Work out the finished part from the listing and answer in its coordinate system (mm). Face numbers are marked on the shaded views. A direction names the side the tool comes from. Round coordinates to 2 decimals unless told otherwise and drop trailing zeros. Order: outer loops, then holes, each group sorted by start corner. A loop starts at its lowest first (then second) coordinate and runs counter-clockwise, first axis right, second up. Notation, with made-up numbers: (3.5, 15.5) - (26.5, 15.5) arc R21 cw to (26.5, 52.5) - close; hole circle Ø10 at (22, 85). An arc over 180 degrees is marked (long way). Answer in a Markdown table with one row per item.
from build123d import *

# Parameters (mm, degrees)
F1_DEPTH  = 6
F3_DEPTH  = 20
F5_DEPTH  = 40
F7_DEPTH  = 60
F9_DEPTH  = 2
F11_DEPTH = 2
F13_DEPTH = 2
F14_R     = 2.25
F15_DEPTH = 8
F16_R     = 2.25
F17_DEPTH = 8
F18_R     = 2.25
F19_DEPTH = 8
F20_R     = 3.75
F21_DEPTH = 2
F22_R     = 3.75
F23_DEPTH = 2
F24_R     = 3.75
F25_DEPTH = 2
F26_SIZE  = 3
F27_W     = 20
F27_H     = 20
F28_DEPTH = 20


with BuildPart() as f1:
    # F0 (on Top) → F1 (new body)
    with BuildSketch(Plane.XY):
        Polygon((0, 66), (0, 0), (66, 0), (66, 26), (26, 26), (26, 66), align=None)
    extrude(amount=F1_DEPTH)

    # F2 (on face) → F3 (join)
    with BuildSketch(Plane.XY.offset(6)):
        Polygon((6, 66), (0, 66), (0, 0), (66, 0), (66, 6), (6, 6), align=None)
    extrude(amount=F3_DEPTH)

    # F4 (on face) → F5 (join)
    with BuildSketch(Plane.XY.offset(26)):
        Polygon((6, 6), (6, 26), (0, 26), (0, 0), (26, 0), (26, 6), align=None)
    extrude(amount=F5_DEPTH)

    # F6 (on face) → F7 (join)
    with BuildSketch(Plane.XY.offset(6)):
        Polygon((13.29, 6), (16, 6), (18.71, 6), (18.71, 8), (13.29, 8), align=None)
        Polygon((6, 18.71), (6, 16), (6, 13.29), (8, 13.29), (8, 18.71), align=None)
    extrude(amount=F7_DEPTH)

    # F8 (on face) → F9 (join)
    with BuildSketch(Plane.XY.offset(6)):
        Polygon((66, 13.29), (66, 16), (66, 18.71), (26, 18.71), (26, 13.29), align=None)
        Polygon((18.71, 66), (16, 66), (13.29, 66), (13.29, 26), (18.71, 26), align=None)
    extrude(amount=F9_DEPTH)

    # F10 (on face) → F11 (join)
    with BuildSketch(Plane(origin=(0, 6, 0), x_dir=(-1, 0, 0), z_dir=(0, 1, 0))):
        Polygon((-66, 18.71), (-66, 16), (-66, 13.29), (-26, 13.29), (-26, 16), (-26, 18.71), align=None)
    extrude(amount=F11_DEPTH)

    # F12 (on face) → F13 (join)
    with BuildSketch(Plane.YZ.offset(6)):
        Polygon((66, 13.29), (66, 16), (66, 18.71), (26, 18.71), (26, 13.29), align=None)
    extrude(amount=F13_DEPTH)

    # F14 (on face) → F15 (cut, through all)
    with BuildSketch(Plane.XZ):
        with Locations((56, 16)):
            Circle(F14_R)
        with Locations((16, 46)):
            Circle(F14_R)
        with Locations((36, 16)):
            Circle(F14_R)
    extrude(amount=-F15_DEPTH, mode=Mode.SUBTRACT)

    # F16 (on face) → F17 (cut, through all)
    with BuildSketch(Plane(origin=(0, 0, 0), x_dir=(0, -1, 0), z_dir=(-1, 0, 0))):
        with Locations((-16, 56)):
            Circle(F16_R)
        with Locations((-46, 16)):
            Circle(F16_R)
        with Locations((-16, 36)):
            Circle(F16_R)
    extrude(amount=-F17_DEPTH, mode=Mode.SUBTRACT)

    # F18 (on face) → F19 (cut, through all)
    with BuildSketch(Plane(origin=(0, 0, 0), x_dir=(1, 0, 0), z_dir=(0, 0, -1))):
        with Locations((46, -16)):
            Circle(F18_R)
        with Locations((16, -56)):
            Circle(F18_R)
        with Locations((16, -36)):
            Circle(F18_R)
    extrude(amount=-F19_DEPTH, mode=Mode.SUBTRACT)

    # F20 (on face) → F21 (cut)
    with BuildSketch(Plane.XZ):
        with Locations((16, 46)):
            Circle(F20_R)
        with Locations((36, 16)):
            Circle(F20_R)
        with Locations((56, 16)):
            Circle(F20_R)
    extrude(amount=-F21_DEPTH, mode=Mode.SUBTRACT)

    # F22 (on face) → F23 (cut)
    with BuildSketch(Plane(origin=(0, 0, 0), x_dir=(0, -1, 0), z_dir=(-1, 0, 0))):
        with Locations((-16, 56)):
            Circle(F22_R)
        with Locations((-46, 16)):
            Circle(F22_R)
        with Locations((-16, 36)):
            Circle(F22_R)
    extrude(amount=-F23_DEPTH, mode=Mode.SUBTRACT)

    # F24 (on face) → F25 (cut)
    with BuildSketch(Plane(origin=(0, 0, 0), x_dir=(1, 0, 0), z_dir=(0, 0, -1))):
        with Locations((16, -56)):
            Circle(F24_R)
        with Locations((46, -16)):
            Circle(F24_R)
        with Locations((16, -36)):
            Circle(F24_R)
    extrude(amount=-F25_DEPTH, mode=Mode.SUBTRACT)

    # F26
    f26_edges = [f1.edges().sort_by_distance(p)[0] for p in [
        (33, 0, 0),
        (0, 33, 0),
        (0, 0, 33),
        (0, 26, 46),
        (0, 46, 26),
        (26, 0, 46),
        (46, 0, 26),
        (0, 13, 66),
        (13, 0, 66),
        (0, 66, 13),
        (13, 66, 0),
        (66, 0, 13),
        (66, 13, 0),
        (46, 26, 0),
        (26, 46, 0),
    ]]
    chamfer(f26_edges, length=F26_SIZE)

    # F27 (on face) → F28 (join)
    with BuildSketch(Plane.XY.offset(6)):
        with Locations((16, 16)):
            Rectangle(F27_W, F27_H)
    extrude(amount=F28_DEPTH)


solid = f1.part
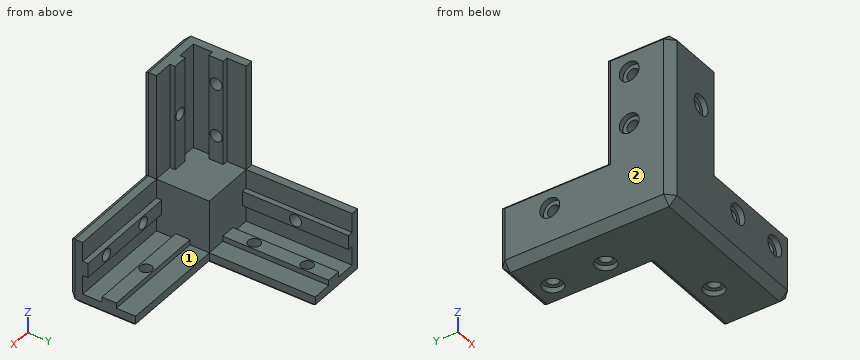
1) Find section C-C, the plane z = 21.5. Give the vertices of the cut face in (x, y), then the cut area to 3 significant figures.
Filled in:
| item | result |
|---|---|
| outline | (0, 3) - (3, 0) - (63, 0) - (66, 3) - (66, 6) - (26, 6) - (26, 26) - (6, 26) - (6, 66) - (3, 66) - (0, 63) - close |
| area | 1,140 mm^2 |
2) Which of the six approach directions +Z, -Z, +X, -X, +Y, -Y give full straight-line access (tool end or side, diameter ignored) to the marked faces 1 and 2?
Filled in:
| item | result |
|---|---|
| face 1 | +Z, +X, +Y |
| face 2 | +Z, -Z, -X, +Y, -Y |
3) Find section A-A, the plane x = 36. Give the vertices of the cut face in (y, z).
Filled in:
| item | result |
|---|---|
| outline | (0, 3) - (3, 0) - (23, 0) - (26, 3) - (26, 6) - (18.71, 6) - (18.71, 8) - (13.29, 8) - (13.29, 6) - (6, 6) - (6, 13.29) - (8, 13.29) - (8, 13.75) - (2, 13.75) - (2, 12.25) - (0, 12.25) - close; (0, 19.75) - (2, 19.75) - (2, 18.25) - (8, 18.25) - (8, 18.71) - (6, 18.71) - (6, 26) - (3, 26) - (0, 23) - close |
4) Find section D-D, the plane y = 24. Give the vertices of the cut face in (x, z).
Filled in:
| item | result |
|---|---|
| outline | (0, 3) - (3, 0) - (23, 0) - (24, 1) - (64, 1) - (66, 3) - (66, 6) - (26, 6) - (26, 26) - (6, 26) - (6, 66) - (3, 66) - (1, 64) - (1, 24) - (0, 23) - close |
5) Find the intervals of material crossed by probe 1 along Y at (x, z) = (16, 0.95); probe 2 along X at (y, z) = (56, 4.3); probe 3 along X at (y, z) = (14.5, 30), in increasing order. Write a range as from..to.
Filled in:
| item | result |
|---|---|
| probe 1 | y = 2.05..32.25, 39.75..52.25, 59.75..63.95 |
| probe 2 | x = 0..13.75, 18.25..26 |
| probe 3 | x = 0..8 |
6) Find section B-B, the plane y = 36. Give the vertices of the cut face in (x, z), then the cut area to 3 significant figures.
Filled in:
| item | result |
|---|---|
| outline | (0, 3) - (3, 0) - (12.25, 0) - (12.25, 2) - (13.75, 2) - (13.75, 8) - (13.29, 8) - (13.29, 6) - (6, 6) - (6, 13.29) - (8, 13.29) - (8, 18.71) - (6, 18.71) - (6, 26) - (3, 26) - (0, 23) - close; (18.25, 2) - (19.75, 2) - (19.75, 0) - (23, 0) - (26, 3) - (26, 6) - (18.71, 6) - (18.71, 8) - (18.25, 8) - close |
| area | 242 mm^2 |
7) Each of these flat-tipped pins is pushed along its axis until it touches: pin 1 (16 mm diameter, centred on x = 20.5, y = 20.5, fed in from +Z); pin 2 (3.5 mm diameter, centred on x = 50, z = 4, fed in from +Y); pin 3 (3.5 mm diameter, centred on x = 21, y = 40.5, fed in from +Z); pin 4 (12 mm diameter, centred on x = 53.5, z = 37, fed in from +Y). Where does it stop, or does it pass through?
Filled in:
| item | result |
|---|---|
| pin 1 | stops at z = 26 |
| pin 2 | stops at y = 26 |
| pin 3 | stops at z = 6 |
| pin 4 | passes through |
